Geometry: final body of the model. Coordinates: model frame, mm. Give positions to 0.01 mm unless a question says otherwise; leave off trailing zeros. Loops run counter-clockwise (first coordinate to the right, second up) from the corner with the lowest first, then second, coordinate; pieces in that order, holes last. Notation, with made-up numbers: (52, 54.25) -> (99, 54.25) arc R16 cw to (99, 79.25) -> close; hole circle Ø6 at (70, -4.75). An arc over 180 degrees is marked (long way). Answer in a Markdown table with one row per item. Add a question column.
from build123d import *

# Parameters (mm, degrees)
BOSS_EXTRUDE1_DEPTH   = 3.175
F_4_CLEARANCE_HOLE1_D = 2.159
F_4_CLEARANCE_HOLE2_D = 2.9464


with BuildPart() as part:
    # Sketch1 → Boss-Extrude1 (new body)
    with BuildSketch(Plane(origin=(0, 0, 0), x_dir=(1, 0, 0), z_dir=(0, 1, 0))):
        with BuildLine():
            Line((20.150112608, -30.9245), (-20.150112608, -30.9245))
            ThreePointArc((-20.150112608, -30.9245), (-32.36664613, -25.86424613), (-37.4269, -13.647712608))
            Line((-37.4269, -13.647712608), (-37.4269, 13.647712608))
            ThreePointArc((-37.4269, 13.647712608), (-32.36664613, 25.86424613), (-20.150112608, 30.9245))
            Line((-20.150112608, 30.9245), (20.150112608, 30.9245))
            ThreePointArc((20.150112608, 30.9245), (32.36664613, 25.86424613), (37.4269, 13.647712608))
            Line((37.4269, 13.647712608), (37.4269, -13.647712608))
            ThreePointArc((37.4269, -13.647712608), (32.36664613, -25.86424613), (20.150112608, -30.9245))
        make_face()
    extrude(amount=BOSS_EXTRUDE1_DEPTH)

    # #4 Clearance Hole1 (through all)
    with Locations(Plane(origin=(0, 3.175, 0), x_dir=(-1, 0, 0), z_dir=(0, 1, 0))):
        with Locations((0, -8), (-8, 0), (0, 8), (8, 0)):
            Hole(F_4_CLEARANCE_HOLE1_D / 2)

    # #4 Clearance Hole2 (through all)
    with Locations(Plane(origin=(0, 3.175, 0), x_dir=(-1, 0, 0), z_dir=(0, 1, 0))):
        with Locations((31.1912, -22.098), (-31.1912, -22.098), (-31.1912, 22.098), (31.1912, 22.098), (34.5, -8.9535), (34.5, 8.9535), (-34.5, 8.9535), (-34.5, -8.9535)):
            Hole(F_4_CLEARANCE_HOLE2_D / 2)


solid = part.part
(1) Cut plane A-A on x = 0. Return the cut outline in (y, z) (1 decimal).
(2) Draft query along Z for faces 1 (the flat face through (0, 2, -30.924)), 2 (the cylindrical face through (30.999, 1.565, -20.637)), 3 (the flat face through (37.427, 2, 0)), 4 (the flat face through (0, 2, 30.924)). Return one class per face: +Z half, -Z half, draft (parallel to the pull), parting line (faces both ways), or undercut.
(3) Cut plane B-B on x = -30.5. Return the cut outline in (y, z) (3 decimals), then the cut area to 3 significant figures.
(4) Cut plane C-C on y = 0.65. State how many separate pieces and enclosed holes the cut face has, then the cut area to 3 significant figures.
(5) Pin query (flat end, axial travel): pin 1 Ø2.5 at (x, z) = (-34.5, 8.95) entering from +Y; pin 2 Ø1 at (y, z) = (1, -22.5) entering from -X. Return the tip coordinate at first contact, or that it passes through.
(6) Material intervals for line 1 along Z through (x, y) = (0, 0.85); line 2 along Z through (x, y) = (-31, 0.45); line 3 along X through (y, z) = (1.1, -9.5), sorted ascending. Write a range as from..to.
Answer list:
| question | item | result |
|---|---|---|
| 1 | outline | (0, -30.9) -> (3.2, -30.9) -> (3.2, -9.1) -> (0, -9.1) -> close; (0, -6.9) -> (3.2, -6.9) -> (3.2, 6.9) -> (0, 6.9) -> close; (0, 9.1) -> (3.2, 9.1) -> (3.2, 30.9) -> (0, 30.9) -> close |
| 2 | face 1 | -Z half |
| 2 | face 2 | undercut |
| 2 | face 3 | draft |
| 2 | face 4 | +Z half |
| 3 | outline | (0, -27.481) -> (3.175, -27.481) -> (3.175, -23.399) -> (0, -23.399) -> close; (0, -20.797) -> (3.175, -20.797) -> (3.175, 20.797) -> (0, 20.797) -> close; (0, 23.399) -> (3.175, 23.399) -> (3.175, 27.481) -> (0, 27.481) -> close |
| 3 | area | 158 mm² |
| 4 | separate pieces | 1 |
| 4 | enclosed holes | 12 |
| 4 | area | 4,300 mm² |
| 5 | pin 1 | passes through |
| 5 | pin 2 | stops at x = -35.27 |
| 6 | line 1 | z = -30.92..-9.08, -6.92..6.92, 9.08..30.92 |
| 6 | line 2 | z = -27.09..-23.56, -20.64..20.64, 23.56..27.09 |
| 6 | line 3 | x = -37.43..-35.87, -33.13..33.13, 35.87..37.43 |
